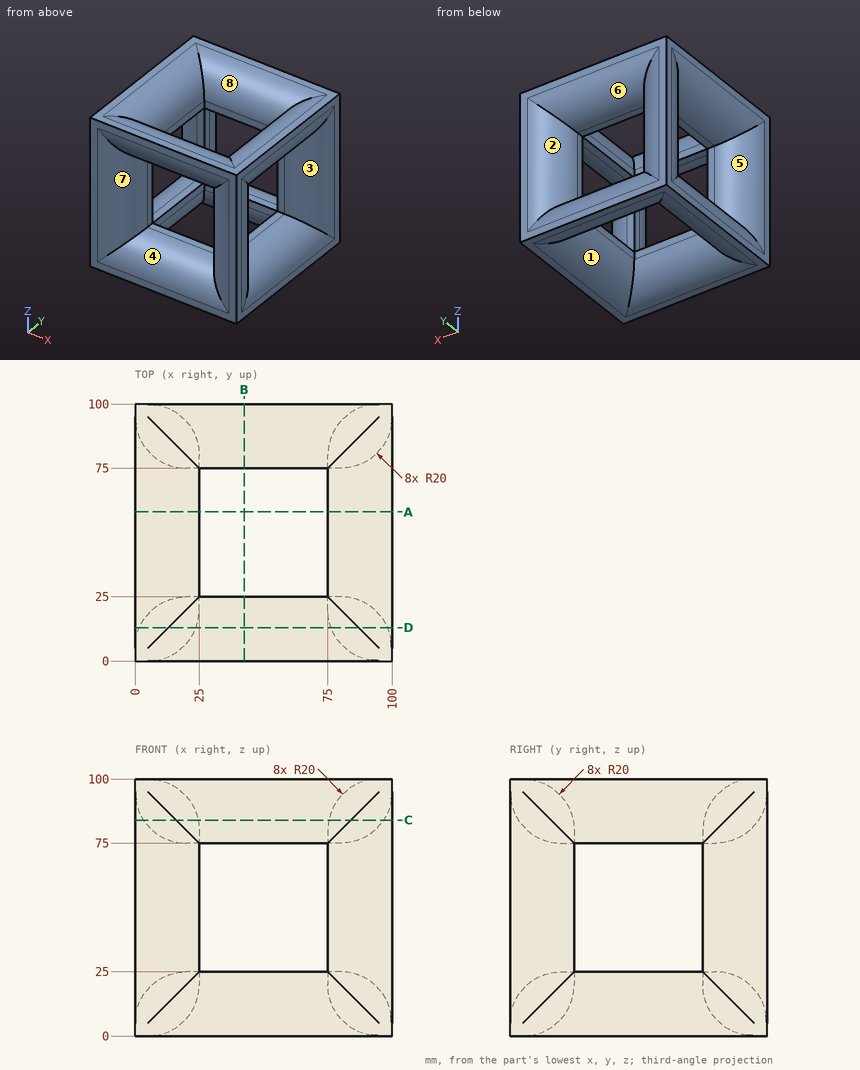
The figure shows three views and two pictorial views of one solid part (mm, origin at its lowest corner). Answer the questions. A direction names the side the tool comes from. Give positions to 0.01 mm unless a question says otherwise; leave off trailing zeros. Write each loop counter-clockwise with the first axis right and the second up, starting at its lowest first coordinate (ties: lowest second). Pieces come first, ordered by that corner, then holes.
Q1. A tool of negligible diameter and unlimited length cuts with its end or side. For the marked faces 1, 2, 3, 4 and 5, from which of +Z, -Z, +X, -X, +Y, -Y can it reach the whole face along a straight path? Write none if from no direction.
Answer:
face 1: -Z
face 2: +Y
face 3: +X
face 4: -Y
face 5: -X
Q2. The part is cut by section A-A on y = 58. Give the vertices of the cut face in (x, z).
Answer:
outline: (0, 0) - (5, 0) arc R20 ccw to (25, 20) - (25, 25) - (20, 25) arc R20 ccw to (0, 5) - close; (0, 95) arc R20 ccw to (20, 75) - (25, 75) - (25, 80) arc R20 ccw to (5, 100) - (0, 100) - close; (75, 20) arc R20 ccw to (95, 0) - (100, 0) - (100, 5) arc R20 ccw to (80, 25) - (75, 25) - close; (75, 75) - (80, 75) arc R20 ccw to (100, 95) - (100, 100) - (95, 100) arc R20 ccw to (75, 80) - close
Q3. The part is cut by section C-C on z = 84. Give the vertices of the cut face in (x, y).
Answer:
outline: (0, 0) - (5, 0) arc R20 ccw to (16, 3.3) - (84, 3.3) arc R20 ccw to (95, 0) - (100, 0) - (100, 5) arc R20 ccw to (96.7, 16) - (96.7, 84) arc R20 ccw to (100, 95) - (100, 100) - (95, 100) arc R20 ccw to (84, 96.7) - (16, 96.7) arc R20 ccw to (5, 100) - (0, 100) - (0, 95) arc R20 ccw to (3.3, 84) - (3.3, 16) arc R20 ccw to (0, 5) - close; hole (24.6, 24.6) - (75.4, 24.6) - (75.4, 75.4) - (24.6, 75.4) - close
Q4. Given pin 1 (5.5 mm diameter, centred on x = 59.5, z = 23, fed in from -Y); pin 2 (3 mm diameter, centred on y = 16, z = 74.5, fed in from -X); pin 3 (12 mm diameter, centred on x = 71, y = 84.5, fed in from +Z), each flat-ended and moving along its own axis, determine where each tip first touches the part or whether it passes through.
Answer:
pin 1: stops at y = 7.06
pin 2: stops at x = 2.4
pin 3: stops at z = 99.49
Q5. Straight lines are drawn through the part: L1, parallel to Y at x = 79, z = 49.5; L2, parallel to X at y = 37, z = 78; L3, parallel to Y at x = 63.5, z = 81. For each, find the intervals that lie inside material, in ascending order.
Answer:
L1: y = 8 to 25, 75 to 92
L2: x = 9.46 to 25, 75 to 90.54
L3: y = 5.72 to 24.97, 75.03 to 94.28
Q6. The part is cut by section D-D on y = 13. Give the vertices of the cut face in (x, z) (3 decimals), and give its area (3 significant figures).
Answer:
outline: (0, 0) - (5, 0) arc R20 ccw to (13, 1.67) - (87, 1.67) arc R20 ccw to (95, 0) - (100, 0) - (100, 5) arc R20 ccw to (98.33, 13) - (98.33, 87) arc R20 ccw to (100, 95) - (100, 100) - (95, 100) arc R20 ccw to (87, 98.33) - (13, 98.33) arc R20 ccw to (5, 100) - (0, 100) - (0, 95) arc R20 ccw to (1.67, 87) - (1.67, 13) arc R20 ccw to (0, 5) - close; hole (23.735, 23.735) - (76.265, 23.735) - (76.265, 76.265) - (23.735, 76.265) - close
area: 6,710 mm2
Q7. For a pull along Y with two mould halves and no side action, classify the marked faces 6, 7 and 8 as released by +Y, released by -Y, zero draft, split by the parting line, or undercut.
Answer:
face 6: released by +Y
face 7: released by -Y
face 8: undercut
